Can you work these out from the drawing? Everything is in mm from the part's minimum corner. Coordinates: 2 decimals unless noted, no trailing zeros. Loops run counter-clockwise (first coordinate to the right, second up) from the corner with the lowest first, then second, coordinate; pieces in that order, holes last. Notation, with made-up numbers: (15.25, -17.5) - (46.25, -17.5) arc R33 ccw to (46.25, 11.5) - close; hole circle Ø2 at (64, 85.5). An arc over 180 degrees is marked (long way). One line per question, with ' | ' between items. Start each with the question number.
1. I want a section at B-B, the plane x = 460. Write out the boundary of the cut face in (y, z).
2. I want a section at C-C, the plane y = 11.75. Write out the boundary of the cut face in (x, z).
3. I want a section at D-D, the plane z = 160. Write out the boundary of the cut face in (x, y).
4. I want a section at A-A, the plane z = 63. Write out the boundary of the cut face in (x, y).
5. Please list where these lines run through material, in increasing order: L1, parallel to X at y = 2.25, z = 15.5; L2, parallel to Z at x = 460, y = 7.5; L3, parallel to X at y = 7, z = 158. Write a range as [from, to].
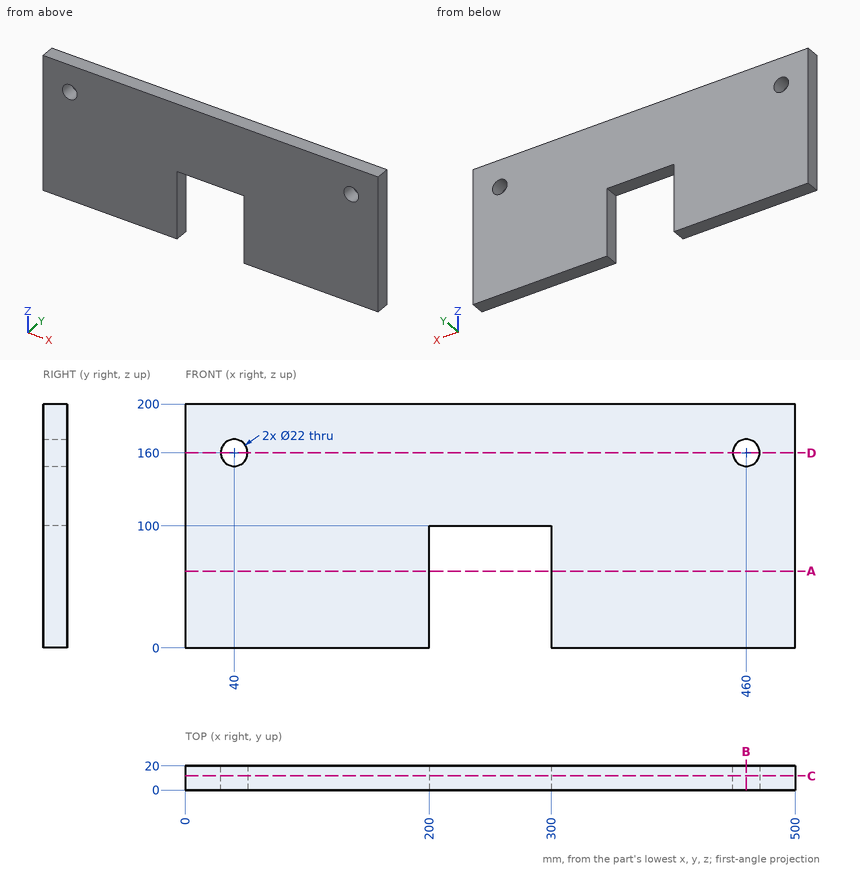
Results are:
1) outline: (0, 0) - (20, 0) - (20, 149) - (0, 149) - close; (0, 171) - (20, 171) - (20, 200) - (0, 200) - close
2) outline: (0, 0) - (200, 0) - (200, 100) - (300, 100) - (300, 0) - (500, 0) - (500, 200) - (0, 200) - close; hole circle Ø22 at (40, 160); hole circle Ø22 at (460, 160)
3) outline: (0, 0) - (29, 0) - (29, 20) - (0, 20) - close; (51, 0) - (449, 0) - (449, 20) - (51, 20) - close; (471, 0) - (500, 0) - (500, 20) - (471, 20) - close
4) outline: (0, 0) - (200, 0) - (200, 20) - (0, 20) - close; (300, 0) - (500, 0) - (500, 20) - (300, 20) - close
5) L1: x = [0, 200], [300, 500] | L2: z = [0, 149], [171, 200] | L3: x = [0, 29.18], [50.82, 449.18], [470.82, 500]
